Check sheet for the modelled part. Datum: model origin and axes. Units: mm. A direction names the side the tool comes from. Round coordinates to 2 decimals unless told otherwise and drop trailing zeros. Write each loop counter-clockwise with the first axis right and the second up, starting at its lowest first coordinate (ties: lowest second). Pieces come first, ordered by that corner, then holes.
Item 1: Material ranges on line 1 along X through (y, z) = (-2, -17.5); line 2 along Z through (x, y) = (14.5, 0.25); line 3 along X through (y, z) = (0, -0.5), recorded low to high.
Item 2: Set-up check for faces 1 (the flat face through (-1, 0, 0.012)), 2 (the flat face through (38, 0, -38.4)): record each of +Z, -Z, +X, -X, +Y, -Y from which the full face is reachable in a straight line by a thin tool's end or side.
Item 3: Section check C-C, the plane x = -13.5. Record the cut outline in (y, z), plus the area to 3 significant figures.
Item 4: Section check B-B, the plane z = -26. Record the cut outline in (x, y).
Item 5: Section check D-D, the plane y = -4. Record the cut outline in (x, z) (1 decimal).
Item 6: Depth check by flat-ended pin: pin 1 (2 mm diameter, centred on y = 3, z = -32.5, fed in from -X); pin 2 (3 mm diameter, centred on x = 11, y = 1, fed in from -Z). Enter the tip coordinate at first touch or a pass-through.
from build123d import *

# Parameters (mm, degrees)
SKETCH1_W                    = 75
SKETCH1_H                    = 10
BOSS_EXTRUDE1_DEPTH          = 1.6
CUT_EXTRUDE1_DEPTH           = 38.865683673
CUT_EXTRUDE1_DEPTH_BACK      = 10
CONVERT_SOLID1_DEPTH         = 0.0125
EDGE_FLANGE1_STRIP_W         = 16.35
EDGE_FLANGE1_STRIP_H         = 1.5875
EDGE_FLANGE1_STRIP_CUT_DEPTH = 10
EDGE_FLANGE1_DEPTH           = 10
FILLET1_R                    = 3


# Read off the part's stored shape, not the designer's step: Convert-Solid1
# Sheet-metal steps are written as plain solids
with BuildPart() as part:
    # Sketch1 → Boss-Extrude1 (new body)
    with BuildSketch(Plane.XY):
        Rectangle(SKETCH1_W, SKETCH1_H)
    extrude(amount=BOSS_EXTRUDE1_DEPTH)

    # Sketch2 → Cut-Extrude1 (cut, two sides: drawn at the far end of the back side and taken through both)
    with BuildSketch(Plane.XY.offset(1.6).offset(-CUT_EXTRUDE1_DEPTH_BACK)):
        Polygon((-37.5, 5), (-37.5, -5), (-27.5, 5), align=None)
    extrude(amount=CUT_EXTRUDE1_DEPTH + CUT_EXTRUDE1_DEPTH_BACK, mode=Mode.SUBTRACT)

    # Convert-Solid1 outline → Convert-Solid1 (cut)
    with BuildSketch(Plane.XY):
        Polygon((37.5, -5), (37.5, 5), (-27.5, 5), (-37.5, -5), align=None)
    extrude(amount=CONVERT_SOLID1_DEPTH, mode=Mode.SUBTRACT)

    # Edge-Flange1 strip (across the edge) → Edge-Flange1 strip cut (cut)
    with BuildSketch(Plane(origin=(37.5, 5, 0.0125), x_dir=(-1, 0, 0), z_dir=(0, -1, 0))):
        with Locations((-3.175, -0.79375)):
            Rectangle(EDGE_FLANGE1_STRIP_W, EDGE_FLANGE1_STRIP_H)
    extrude(amount=EDGE_FLANGE1_STRIP_CUT_DEPTH, mode=Mode.SUBTRACT)

    # Edge-Flange1 section (across the edge) → Edge-Flange1 (add)
    with BuildSketch(Plane(origin=(37.5, 5, 0.0125), x_dir=(-1, 0, 0), z_dir=(0, -1, 0))):
        with BuildLine():
            Line((-1.5875, 5), (-1.5875, 38.4125))
            Line((-1.5875, 38.4125), (0, 38.4125))
            Line((0, 38.4125), (0, 5))
            ThreePointArc((0, 5), (1.464466094, 1.464466094), (5, 0))
            Line((5, 0), (5, -1.5875))
            ThreePointArc((5, -1.5875), (0.341934079, 0.341934079), (-1.5875, 5))
        make_face()
    extrude(amount=EDGE_FLANGE1_DEPTH)

    # Fillet1
    fillet1_edges = [part.edges().sort_by_distance(p)[0] for p in [
        (38.29375, 5, -38.4),
        (38.29375, -5, -38.4),
        (-37.5, -5, 0.80625),
        (-27.5, 5, 0.80625),
    ]]
    fillet(fillet1_edges, radius=FILLET1_R)


solid = part.part
Values found:
1. line 1: x = 37.5 to 39.09
1. line 2: z = 0.01 to 1.6
1. line 3: x = 34.71 to 37.32
2. face 1: -Z, -X, +Y, -Y
2. face 2: -Z, +X, -X, +Y, -Y
3. outline: (-5, 0.01) - (5, 0.01) - (5, 1.6) - (-5, 1.6) - close
3. area: 15.9 mm2
4. outline: (37.5, -5) - (39.09, -5) - (39.09, 5) - (37.5, 5) - close
5. outline: (-32.5, 0) - (32.5, 0) arc R5 cw to (37.5, -5) - (37.5, -37.6) - (39.1, -37.6) - (39.1, -5) arc R6.6 ccw to (32.5, 1.6) - (-32.5, 1.6) - close
6. pin 1: stops at x = 37.5
6. pin 2: stops at z = 0.01
